from build123d import *

# Parameters (mm, degrees)
F0_W     = 76.2
F0_H     = 76.2
F1_DEPTH = 9.525
F2_R     = 31.75
F3_DEPTH = 2.54


with BuildPart() as f1:
    # F0 (on Top) → F1 (new body)
    with BuildSketch(Plane.XY):
        Rectangle(F0_W, F0_H)
    extrude(amount=F1_DEPTH)

    # F2 (on face) → F3 (cut)
    with BuildSketch(Plane.XY.offset(9.525)):
        Circle(F2_R)
        with BuildLine():
            ThreePointArc((29.8215182706, 4.5225495338), (30.0771337654, 2.2676928157), (30.1625, 0))
            ThreePointArc((30.1625, 0), (24.913715506, -17.0024464691), (10.9941163492, -28.0874671687))
            ThreePointArc((10.9941163492, -28.0874671687), (0, -30.1625), (-10.9941163492, -28.0874671687))
            ThreePointArc((-10.9941163492, -28.0874671687), (-26.1214912416, -15.08125), (-29.8215182706, 4.5225495338))
            ThreePointArc((-29.8215182706, 4.5225495338), (-26.1214912416, 15.08125), (-18.8274019215, 23.5649176349))
            ThreePointArc((-18.8274019215, 23.5649176349), (0, 30.1625), (18.8274019215, 23.5649176349))
            ThreePointArc((18.8274019215, 23.5649176349), (26.1214912416, 15.08125), (29.8215182706, 4.5225495338))
        make_face(mode=Mode.SUBTRACT)
        with BuildLine():
            Line((6.1911249981, 1.4115492405), (28.2472801431, 4.3152971525))
            ThreePointArc((28.2472801431, 4.3152971525), (24.7466759131, 14.2875), (17.8607970305, 22.3052136155))
            Line((17.8607970305, 22.3052136155), (4.318, 4.6558969061))
            ThreePointArc((4.318, 4.6558969061), (0, 6.35), (-4.318, 4.6558969061))
            Line((-4.318, 4.6558969061), (-17.8607970305, 22.3052136155))
            ThreePointArc((-17.8607970305, 22.3052136155), (-24.7466759131, 14.2875), (-28.2472801431, 4.3152971525))
            Line((-28.2472801431, 4.3152971525), (-6.1911249981, 1.4115492405))
            ThreePointArc((-6.1911249981, 1.4115492405), (-5.499261314, -3.175), (-1.8731249981, -6.0674461466))
            Line((-1.8731249981, -6.0674461466), (-10.3864831126, -26.620510768))
            ThreePointArc((-10.3864831126, -26.620510768), (0, -28.575), (10.3864831126, -26.620510768))
            Line((10.3864831126, -26.620510768), (1.8731249981, -6.0674461466))
            ThreePointArc((1.8731249981, -6.0674461466), (5.499261314, -3.175), (6.1911249981, 1.4115492405))
        make_face()
    extrude(amount=-F3_DEPTH, mode=Mode.SUBTRACT)


solid = f1.part
Check sheet for the modelled part. Datum: model origin and axes. Units: mm. A direction names the side the tool comes from. Give positions to 0.01 mm unless a question says otherwise; leave off trailing zeros. Loops run counter-clockwise (first coordinate to the right, second up) from the corner with the lowest first, then second, coordinate; pieces in that order, holes last. Notation, with made-up numbers: M 73.5,23.25 L 98.5,23.25 A33 ccw 98.5,52.25 Z; hole C 37,76 d8. An arc over 180 degrees is marked long. Answer as a JSON object with one key per item and string values. Group by question number.
Q1. Release check for a two-part mould opening along X. For faces 3 (the flat face through (0, 7, 9.525)), 4 (the cylindrical face through (24.82, 14.16, 8.27)), 5 (the flat face through (-38.1, -1, 5)) record: released by +X, released by -X, zero draft, split by the parting line, or undercut.
Q2. Cross-section at C-C on x = 27. Record the cut outline in (y, z) (3 decimals).
Q3. Material ranges on line 1 along X through (y, z) = (23, 8); line 2 along Z through (x, y) = (12, 3) (3 decimals), recorded low to high. Write a range as [from, to].
Q4. Cross-section at B-B on y = 28.5. Record the cut outline in (x, z) (3 decimals), then the cut area to 3 significant figures.
Q5. Access from +Z, -Z, +X, -X, +Y, -Y to the whole of each face (thin tool, end or side, straight path). Record for faces 1 (the flat face through (-1, 38.1, 5)), 2 (the cylindrical face through (0.07, 6.35, 8.27)).
Evaluation:
{
 "1": {"face 3": "zero draft", "face 4": "undercut", "face 5": "released by -X"},
 "2": {"outline": "M -38.1,0 L 38.1,0 L 38.1,9.525 L 16.705,9.525 L 16.705,6.985 L 13.445,6.985 L 13.445,9.525 L 9.356,9.525 L 9.356,6.985 L 4.151,6.985 L 4.151,9.525 L -13.445,9.525 L -13.445,6.985 L -16.705,6.985 L -16.705,9.525 L -38.1,9.525 Z"},
 "3": {"line 1": "x = [-38.1, -21.89], [-19.51, 19.51], [21.89, 38.1]", "line 2": "z = [0, 6.985]"},
 "4": {"outline": "M -38.1,0 L 38.1,0 L 38.1,9.525 L 13.993,9.525 L 13.993,6.985 L 9.876,6.985 L 9.876,9.525 L -9.876,9.525 L -9.876,6.985 L -13.993,6.985 L -13.993,9.525 L -38.1,9.525 Z", "area": "705 mm2"},
 "5": {"face 1": "+Z, -Z, +X, -X, +Y", "face 2": "+Z"}
}
